Check sheet for the modelled part. Datum: model origin and axes. Units: mm. A direction names the side the tool comes from. Round coordinates to 2 decimals unless told otherwise and drop trailing zeros. Write each loop counter-clockwise with the first axis right and the second up, starting at its lowest first coordinate (ties: lowest second). Pieces come first, ordered by that corner, then holes. Notation, with made-up numbers: (25, -21.5) -> (58, -21.5) arc R16 ccw to (58, -12.5) -> close; hole circle Ø3 at (40.25, 77). An arc over 180 degrees is marked (long way). Write item = value, one per line.
from build123d import *

# Parameters (mm, degrees)
F1_DEPTH = 6
F2_R     = 1.5
F3_DEPTH = 25


with BuildPart() as f1:
    # F0 (on Right) → F1 (new body)
    with BuildSketch(Plane.YZ):
        Polygon((-9, 0), (0, 0), (0, 6), (-3, 6), (-3, 3), (-9, 3), align=None)
    extrude(amount=F1_DEPTH)

    # F2 (on face) → F3 (cut)
    with BuildSketch(Plane.XY.offset(3)):
        with Locations((3, -7)):
            Circle(F2_R)
    extrude(amount=-F3_DEPTH, mode=Mode.SUBTRACT)


solid = f1.part
(1) Sectioned sample at D-D on x = 4.9. Enter the section's corners in (y, z).
Worked answers:
outline = (-9, 0) -> (0, 0) -> (0, 6) -> (-3, 6) -> (-3, 3) -> (-9, 3) -> close
(2) Go/stop test with flat-tipped pins: P1, Ø1.5, axis at x = 3, y = -6, coming from the +Z side; P2, Ø1.5, axis at x = 1.5, z = 4, coming from the -Y side; P3, Ø1.5, axis at x = 1, y = -5.5, coming from the -Z side. Record where each tip stops, or that it passes through.
Worked answers:
P1 = 3
P2 = -3
P3 = 0
(3) Sectioned sample at C-C on z = 1.2. Enter the section's corners in (x, y), then the cut area to 3 significant figures.
Worked answers:
outline = (0, -9) -> (6, -9) -> (6, 0) -> (0, 0) -> close; hole circle Ø3 at (3, -7)
area = 46.9 mm²
(4) Sectioned sample at B-B on y = -7. Enter the section's corners in (x, z), then the cut area to 3 significant figures.
Worked answers:
outline = (0, 0) -> (1.5, 0) -> (1.5, 3) -> (0, 3) -> close; (4.5, 0) -> (6, 0) -> (6, 3) -> (4.5, 3) -> close
area = 9.00 mm²
(5) Release check for a two-part mould opening along X. For faces 1 (the flat face through (3, -5, 0)), 2 (the flat face through (6, -4, 2)), 3 (the cylindrical face through (2.675, -8.464, 1.521)) record: pulls with the +X half, pulls with the -X half, needs draft (parallel to the pull), parting line crosses it, or undercut.
Worked answers:
face_1 = needs draft
face_2 = pulls with the +X half
face_3 = undercut
(6) Sectioned sample at A-A on x = 3. Enter the section's corners in (y, z).
Worked answers:
outline = (-9, 0) -> (-8.5, 0) -> (-8.5, 3) -> (-9, 3) -> close; (-5.5, 0) -> (0, 0) -> (0, 6) -> (-3, 6) -> (-3, 3) -> (-5.5, 3) -> close
(7) Access from +Z, -Z, +X, -X, +Y, -Y to the whole of each face (thin tool, end or side, straight path). Record for faces 4 (the flat face through (3, -5, 3)), 5 (the flat face through (3, -9, 2)).
Worked answers:
face_4 = +Z, +X, -X, -Y
face_5 = +Z, -Z, +X, -X, -Y
(8) Material ranges on L1, parallel to Y at x = 3, z = 0.85; L2, parallel to Y at x = 4.3, z = 4.2; L3, parallel to Z at x = 1.75, y = -5.25, recorded low to high. Write a range as [from, to].
Worked answers:
L1 = [-9, -8.5], [-5.5, 0]
L2 = [-3, 0]
L3 = [0, 3]
